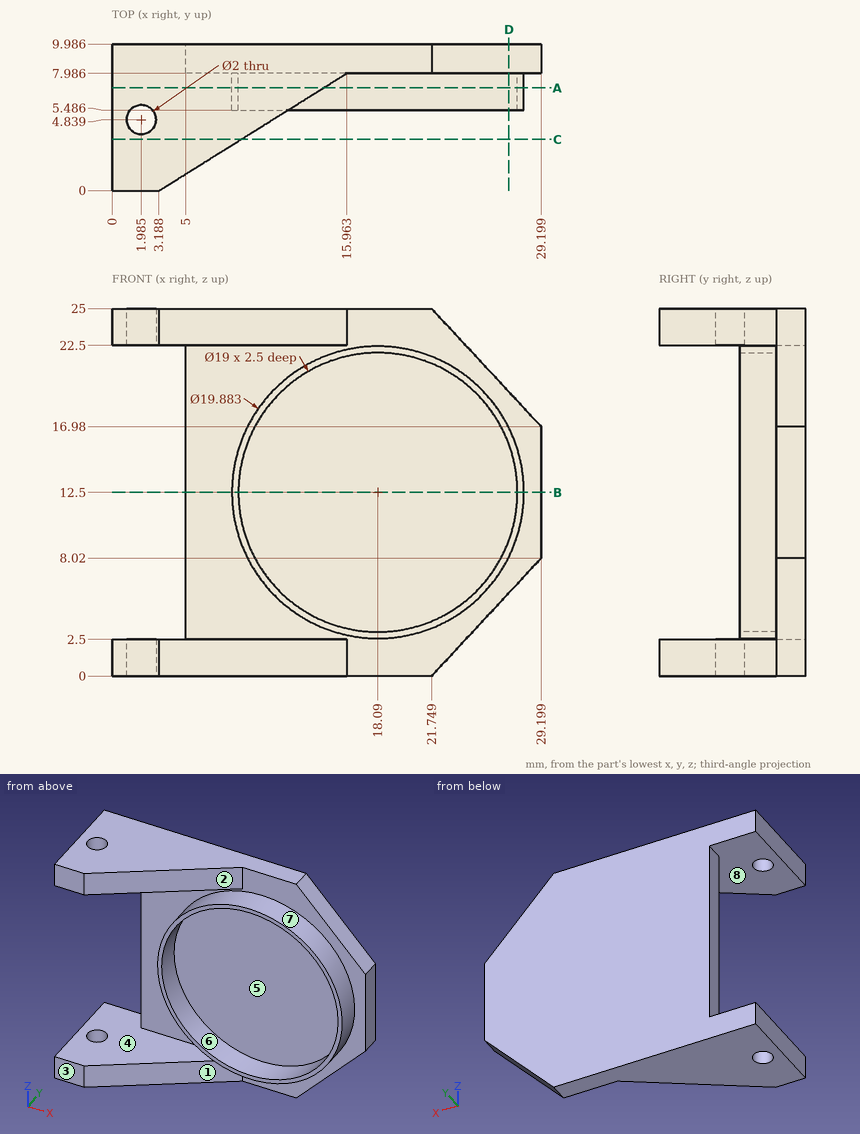
Input: dimensioned drawing with shaded views. Units: mm. Origin: part minimum x, y, z. A direction names the side the tool comes from. Round coordinates to 2 decimals unless told otherwise and drop trailing zeros. Loops run counter-clockwise (first coordinate to the right, second up) from the corner with the lowest first, then second, coordinate; pieces in that order, holes last. Notation, with made-up numbers: (75, 18.5) -> (97, 18.5) arc R20 ccw to (97, 40.5) -> close; hole circle Ø11 at (45.25, 52). An arc over 180 degrees is marked (long way). Answer as a JSON object with one key per item and string values. Group by question number.
1) Ray query, L1, parallel to Z at x = 7.5, y = 7.5; L2, parallel to X at y = 6, z = 12.5; L3, parallel to Y at x = 23, z = 1.5. Return the intervals inside material, ascending.
2) Draft query along X for the marked faces 6, 7 and 8. Return one class per face: +X half, -X half, draft (parallel to the pull), parting line (faces both ways), or undercut.
3) Pin query (flat end, axial travel): pin 1 (4 mm diameter, centred on x = 4.5, z = 12.5, fed in from -Y); pin 2 (10 mm diameter, centred on x = 15, z = 16.5, fed in from -Y); pin 3 (2 mm diameter, centred on y = 9, z = 9, fed in from -X). Return the tip coordinate at first contact, or that it passes through.
4) Section query A-A on y = 7. Output: boundary loops of the cut face in (x, z) (1 decimal).
5) Section query C-C on y = 3.5. Output: boundary loops of the cut face in (x, z).
6) Reachability of the marked faces 1, 2, 3, 4 and 5 from +Z, -Z, +X, -X, +Y, -Y: full face, straight path, thin tool, end or side. Return the list, or none.
7) Section query D-D on x = 27. Output: boundary loops of the cut face in (y, z) (1 decimal).
8) Section query B-B on z = 12.5. Output: boundary loops of the cut face in (x, y).
Reply:
{
 "1": {"L1": "z = 0 to 2.5, 22.5 to 25", "L2": "x = 8.15 to 8.59, 27.59 to 28.03", "L3": "y = 7.99 to 9.99"},
 "2": {"face 6": "undercut", "face 7": "parting line", "face 8": "draft"},
 "3": {"pin 1": "stops at y = 7.99", "pin 2": "stops at y = 5.49", "pin 3": "stops at x = 5"},
 "4": {"outline": "(0, 0) -> (14.4, 0) -> (14.4, 2.5) -> (0, 2.5) -> close; (0, 22.5) -> (14.4, 22.5) -> (14.4, 25) -> (0, 25) -> close; circle Ø19.9 at (18.1, 12.5); hole circle Ø19 at (18.1, 12.5)"},
 "5": {"outline": "(0, 0) -> (8.79, 0) -> (8.79, 2.5) -> (0, 2.5) -> close; (0, 22.5) -> (8.79, 22.5) -> (8.79, 25) -> (0, 25) -> close"},
 "6": {"face 1": "-Z, +X, -Y", "face 2": "+Z, +X, -Y", "face 3": "+Z, -Z, +X, -X, -Y", "face 4": "-X, -Y", "face 5": "-Y"},
 "7": {"outline": "(5.5, 8.1) -> (8, 8.1) -> (8, 5.7) -> (10, 5.7) -> (10, 19.3) -> (8, 19.3) -> (8, 16.9) -> (5.5, 16.9) -> (5.5, 15.8) -> (8, 15.8) -> (8, 9.2) -> (5.5, 9.2) -> close"},
 "8": {"outline": "(5, 7.99) -> (8.15, 7.99) -> (8.15, 5.49) -> (8.59, 5.49) -> (8.59, 7.99) -> (27.59, 7.99) -> (27.59, 5.49) -> (28.03, 5.49) -> (28.03, 7.99) -> (29.2, 7.99) -> (29.2, 9.99) -> (5, 9.99) -> close"}
}
